Check sheet for the drawn part. Datum: minimum x, y, z corner. Units: mm. A direction names the side the tool comes from. Give positions to 0.01 mm unless a question says otherwise; leave off trailing zeros. Loops run counter-clockwise (first coordinate to the right, second up) from the corner with the lowest first, then second, coordinate; pieces in that order, holes last.
1. Release check for a two-part mould opening along X. For the marked faces 1, 2, 3 and 4 record: +X half, -X half, draft (parallel to the pull), parting line (faces both ways), or undercut.
2. Cross-section at B-B, the plane x = 33. Record the cut outline in (y, z) (1 decimal).
3. Material ranges on L1, parallel to X at y = 5, z = 43; L2, parallel to Z at x = 35, y = 4; L3, parallel to X at y = 1.25, z = 5, recorded low to high.
4. Tool access check on the marked faces 5 and 6. Record the directions out of +Z, -Z, +X, -X, +Y, -Y that give a thin tool (end or side, any length) a straight path to the whole face; none if there is none.
5. Cross-section at A-A, the plane z = 27. Record the cut outline in (x, y) (1 decimal).
6. Go/stop test with a flat-tipped pin: pin 1 Ø1.4 at (x, z) = (15.45, 68) entering from -Y. Record where the tip stops, or that it passes through.
7. Cross-section at C-C, the plane y = 5.5. Record the cut outline in (x, z) (1 decimal), plus the area to 3 significant figures.
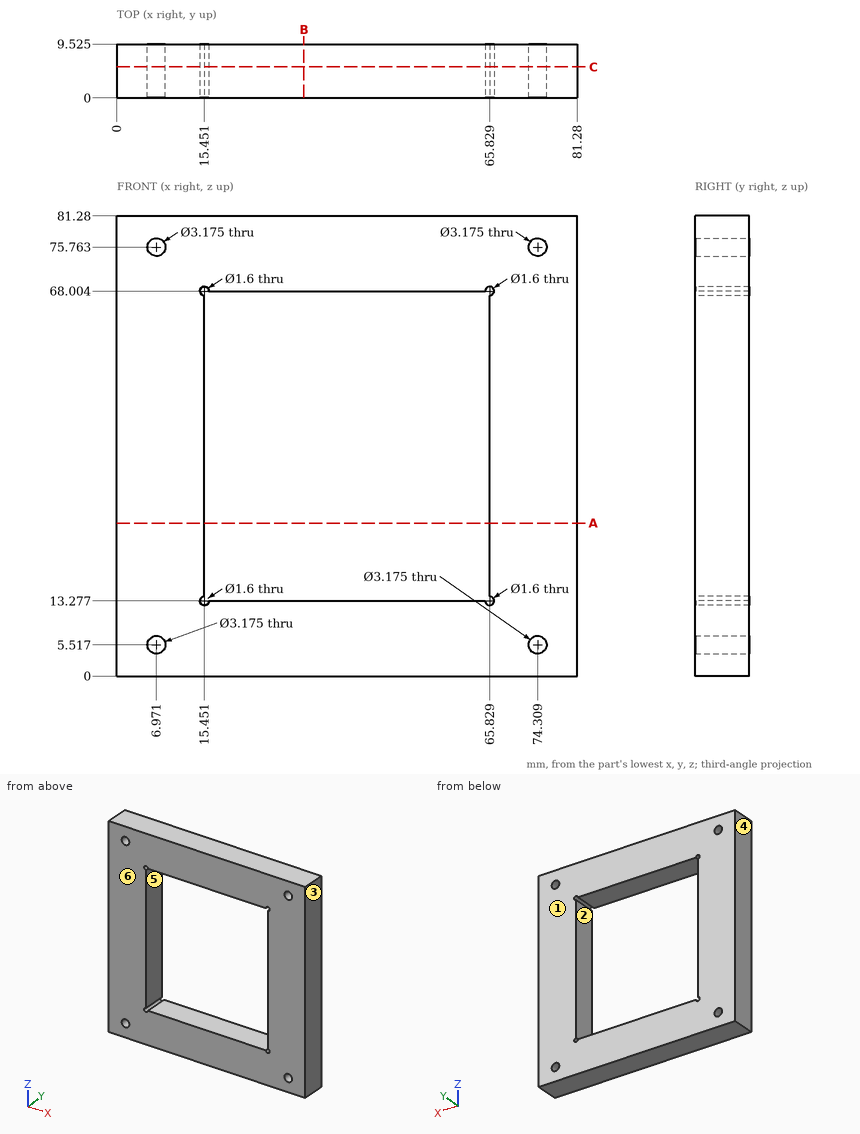
Result:
1. face 1: draft
1. face 2: undercut
1. face 3: +X half
1. face 4: -X half
2. outline: (0, 0) - (9.5, 0) - (9.5, 13.3) - (0, 13.3) - close; (0, 68) - (9.5, 68) - (9.5, 81.3) - (0, 81.3) - close
3. L1: x = 0 to 15.45, 65.83 to 81.28
3. L2: z = 0 to 13.28, 68 to 81.28
3. L3: x = 0 to 5.47, 8.47 to 72.81, 75.81 to 81.28
4. face 5: +Y, -Y
4. face 6: +Z, -Z, +X, -X, -Y
5. outline: (0, 0) - (15.5, 0) - (15.5, 9.5) - (0, 9.5) - close; (65.8, 0) - (81.3, 0) - (81.3, 9.5) - (65.8, 9.5) - close
6. pin 1: passes through
7. outline: (0, 0) - (81.3, 0) - (81.3, 81.3) - (0, 81.3) - close; hole circle Ø3.2 at (7, 5.5); hole circle Ø3.2 at (7, 75.8); hole (15.5, 14.1) arc R0.8 ccw (long way) to (16.3, 13.3) - (65, 13.3) arc R0.8 ccw (long way) to (65.8, 14.1) - (65.8, 67.2) arc R0.8 ccw (long way) to (65, 68) - (16.3, 68) arc R0.8 ccw (long way) to (15.5, 67.2) - close; hole circle Ø3.2 at (74.3, 5.5); hole circle Ø3.2 at (74.3, 75.8)
7. area: 3,810 mm2
